Could you check a few things on this model? Use its own coordinates, in mm. Give positions to 0.01 mm unless a question says otherwise; leave off trailing zeros. Write each loop counter-clockwise with the first axis right and the second up, starting at its lowest first coordinate (ties: lowest second). Pieces come first, ordered by that corner, then holes. Notation, with made-up numbers: M 27,77 L 77,77 A35 ccw 77,116 Z; hole C 25,2.25 d11. An arc over 180 degrees is marked long. Use one line per item in the form item = value.
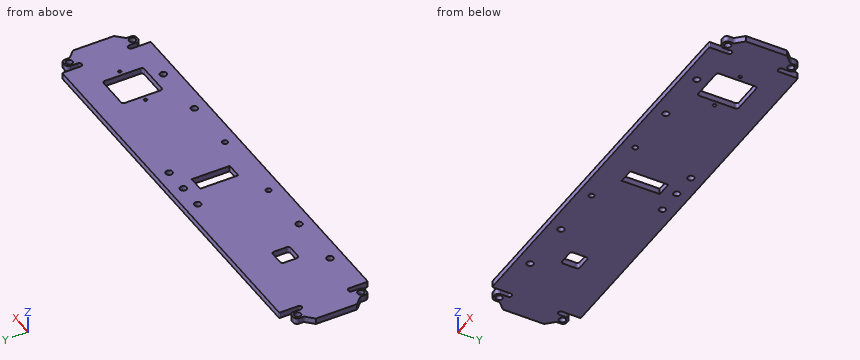
from build123d import *

# Parameters (mm, degrees)
BASE_FLANGE1_DEPTH         = 4.7625
CUT_EXTRUDE1_DEPTH         = 348.163767416
CUT_EXTRUDE2_DEPTH         = 348.163767416
SKETCH20_W                 = 12
SKETCH20_H                 = 30
CUT_EXTRUDE5_DEPTH         = 348.163767416
F_5_2_5_2_DIAMETER_HOLE1_D = 5.2
F_4_2_4_2_DIAMETER_HOLE1_D = 4.2
F_2_5_2_5_DIAMETER_HOLE1_D = 2.5


# Sheet-metal steps are written as plain solids
with BuildPart() as part:
    # Sketch11 → Base-Flange1 (new body)
    with BuildSketch(Plane(origin=(0, 0, 0), x_dir=(-1, 0, 0), z_dir=(0, 0, -1))):
        with BuildLine():
            Line((-17.976164198, 1), (-17.976164198, 14.75465548))
            ThreePointArc((-17.976164198, 14.75465548), (-15.991789198, 16.73903048), (-14.007414198, 14.75465548))
            Line((-14.007414198, 14.75465548), (-14.007414198, 9))
            ThreePointArc((-14.007414198, 9), (-13.128734542, 6.878679656), (-11.007414198, 6))
            Line((-11.007414198, 6), (-9, 6))
            ThreePointArc((-9, 6), (-6.878679657, 6.878679656), (-6, 9))
            Line((-6, 9), (-6, 11.917075442))
            ThreePointArc((-6, 11.917075442), (-5.848948447, 12.676462879), (-5.418790019, 13.320240461))
            Line((-5.418790019, 13.320240461), (0, 18.73903048))
            Line((0, 18.73903048), (0, 51.26096952))
            Line((0, 51.26096952), (-5.418790019, 56.679759539))
            ThreePointArc((-5.418790019, 56.679759539), (-5.848948447, 57.323537121), (-6, 58.082924558))
            Line((-6, 58.082924558), (-6, 61))
            ThreePointArc((-6, 61), (-6.878679657, 63.121320343), (-9, 64))
            Line((-9, 64), (-11.007414198, 64))
            ThreePointArc((-11.007414198, 64), (-13.128734542, 63.121320343), (-14.007414198, 61))
            Line((-14.007414198, 61), (-14.007414198, 55.24534452))
            ThreePointArc((-14.007414198, 55.24534452), (-15.991789198, 53.26096952), (-17.976164198, 55.24534452))
            Line((-17.976164198, 55.24534452), (-17.976164198, 69))
            ThreePointArc((-17.976164198, 69), (-18.269057417, 69.707106781), (-18.976164198, 70))
            Line((-18.976164198, 70), (-321.023835802, 70))
            ThreePointArc((-321.023835802, 70), (-321.730942583, 69.707106781), (-322.023835802, 69))
            Line((-322.023835802, 69), (-322.023835802, 55.24534452))
            ThreePointArc((-322.023835802, 55.24534452), (-322.605045783, 53.842179501), (-324.008210802, 53.26096952))
            Line((-324.008210802, 53.26096952), (-324.039460804, 53.26096952))
            ThreePointArc((-324.039460804, 53.26096952), (-325.442625823, 53.842179501), (-326.023835804, 55.24534452))
            Line((-326.023835804, 55.24534452), (-326.023835804, 61))
            ThreePointArc((-326.023835804, 61), (-326.90251546, 63.121320343), (-329.023835804, 64))
            Line((-329.023835804, 64), (-331, 64))
            ThreePointArc((-331, 64), (-333.121320344, 63.121320343), (-334, 61))
            Line((-334, 61), (-334, 58.082924558))
            ThreePointArc((-334, 58.082924558), (-334.151051553, 57.323537121), (-334.581209981, 56.679759539))
            Line((-334.581209981, 56.679759539), (-340, 51.26096952))
            Line((-340, 51.26096952), (-340, 18.73903048))
            Line((-340, 18.73903048), (-334.581209981, 13.320240461))
            ThreePointArc((-334.581209981, 13.320240461), (-334.151051553, 12.676462879), (-334, 11.917075442))
            Line((-334, 11.917075442), (-334, 9))
            ThreePointArc((-334, 9), (-333.121320344, 6.878679656), (-331, 6))
            Line((-331, 6), (-329.023835804, 6))
            ThreePointArc((-329.023835804, 6), (-326.90251546, 6.878679656), (-326.023835804, 9))
            Line((-326.023835804, 9), (-326.023835804, 14.75465548))
            ThreePointArc((-326.023835804, 14.75465548), (-325.442625823, 16.157820499), (-324.039460804, 16.73903048))
            Line((-324.039460804, 16.73903048), (-324.008210802, 16.73903048))
            ThreePointArc((-324.008210802, 16.73903048), (-322.605045783, 16.157820499), (-322.023835802, 14.75465548))
            Line((-322.023835802, 14.75465548), (-322.023835802, 1))
            ThreePointArc((-322.023835802, 1), (-321.730942583, 0.292893219), (-321.023835802, 0))
            Line((-321.023835802, 0), (-18.976164198, 0))
            ThreePointArc((-18.976164198, 0), (-18.269057417, 0.292893219), (-17.976164198, 1))
        make_face()
    extrude(amount=-BASE_FLANGE1_DEPTH)

    # Sketch16 → Cut-Extrude1 (cut, through all)
    with BuildSketch(Plane(origin=(0, 0, 0), x_dir=(-1, 0, 0), z_dir=(0, 0, -1))):
        with BuildLine():
            Line((-274, 50.597720146), (-298, 50.597720146))
            ThreePointArc((-298, 50.597720146), (-299.414213562, 50.011933709), (-300, 48.597720146))
            Line((-300, 48.597720146), (-300, 20.597720146))
            ThreePointArc((-300, 20.597720146), (-299.414213562, 19.183506584), (-298, 18.597720146))
            Line((-298, 18.597720146), (-274, 18.597720146))
            ThreePointArc((-274, 18.597720146), (-272.585786438, 19.183506584), (-272, 20.597720146))
            Line((-272, 20.597720146), (-272, 48.597720146))
            ThreePointArc((-272, 48.597720146), (-272.585786438, 50.011933709), (-274, 50.597720146))
        make_face()
    extrude(amount=-CUT_EXTRUDE1_DEPTH, mode=Mode.SUBTRACT)

    # Sketch17 → Cut-Extrude2 (cut, through all)
    with BuildSketch(Plane(origin=(0, 0, 0), x_dir=(-1, 0, 0), z_dir=(0, 0, -1))):
        with BuildLine():
            Line((-64.5, 30), (-64.5, 40))
            ThreePointArc((-64.5, 40), (-65.085786438, 41.414213562), (-66.5, 42))
            Line((-66.5, 42), (-76.5, 42))
            ThreePointArc((-76.5, 42), (-77.914213563, 41.414213562), (-78.5, 40))
            Line((-78.5, 40), (-78.5, 30))
            ThreePointArc((-78.5, 30), (-77.914213563, 28.585786438), (-76.5, 28))
            Line((-76.5, 28), (-66.5, 28))
            ThreePointArc((-66.5, 28), (-65.085786438, 28.585786438), (-64.5, 30))
        make_face()
    extrude(amount=-CUT_EXTRUDE2_DEPTH, mode=Mode.SUBTRACT)

    # Sketch20 → Cut-Extrude5 (cut, through all)
    with BuildSketch(Plane.XY.offset(4.7625)):
        with Locations((170, 35)):
            Rectangle(SKETCH20_W, SKETCH20_H)
    extrude(amount=-CUT_EXTRUDE5_DEPTH, mode=Mode.SUBTRACT)

    # Ø5.2 (5.2) Diameter Hole1 (through all)
    with Locations(Plane.XY.offset(4.7625)):
        with Locations((170, 60), (330, 60), (10, 10), (10, 60), (330, 10), (150, 60), (190, 60), (53.333333333, 10), (96.666666667, 10), (243.333333333, 10), (286.666666667, 10)):
            Hole(F_5_2_5_2_DIAMETER_HOLE1_D / 2)

    # Ø4.2 (4.2) Diameter Hole1 (through all)
    with Locations(Plane(origin=(0, 0, 0), x_dir=(-1, 0, 0), z_dir=(0, 0, -1))):
        with Locations((-200.5, 10), (-139.5, 10)):
            Hole(F_4_2_4_2_DIAMETER_HOLE1_D / 2)

    # Ø2.5 (2.5) Diameter Hole1 (through all)
    with Locations(Plane(origin=(0, 0, 0), x_dir=(-1, 0, 0), z_dir=(0, 0, -1))):
        with Locations((-304, 34.597720146), (-268, 34.597720146)):
            Hole(F_2_5_2_5_DIAMETER_HOLE1_D / 2)


solid = part.part
1) I want a section at B-B, the plane z = 1.1. Count the separate pieces of the cut face and the enclosed holes in it, plus the area to 3 significant figures.
Checked values:
separate_pieces = 1
enclosed_holes = 18
area = 21,200 mm2
2) If I drill on L1, parallel to X at y = 48.5, z = 0.4; L2, parallel to X at y = 37.5, z = 2.25; L3, parallel to X at y = 63.5, z = 4.2, over which ranges is the centre line in solid material (lowest first)?
Checked values:
L1 = 0 to 164, 176 to 272, 300 to 340
L2 = 0 to 64.5, 78.5 to 164, 176 to 272, 300 to 340
L3 = 7.34 to 12.67, 17.98 to 322.02, 327.37 to 332.66
3) I want a section at A-A, the plane y = 23.5. Please give me the cut outline in (x, z).
Checked values:
outline = M 0,0 L 164,0 L 164,4.76 L 0,4.76 Z; M 176,0 L 272,0 L 272,4.76 L 176,4.76 Z; M 300,0 L 340,0 L 340,4.76 L 300,4.76 Z
4) For pin 1 Ø2.5 at (y, z) = (7.5, 1.5) entering from +X; pin 2 Ø2 at (y, z) = (58.5, 3.5) entering from -X; pin 3 Ø1.4 at (y, z) = (11, 2.5) entering from -X, each with a flat end and sliding along its axis, tell me the tip position at first contact or that it passes through.
Checked values:
pin_1 = 333.99
pin_2 = 5.91
pin_3 = 6
